from build123d import *

# Parameters (mm, degrees)
SKETCH3_W           = 241.3
SKETCH3_H           = 241.3
SKETCH3_R           = 4.25
BOSS_EXTRUDE1_DEPTH = 12.7
SKETCH4_R           = 7.9375
CUT_EXTRUDE1_DEPTH  = 172.096858533
FILLET1_R           = 12.7
SKETCH5_R           = 7.9375
SKETCH5_R_2         = 10.99947
BOSS_EXTRUDE2_DEPTH = 25.4


with BuildPart() as part:
    # Sketch3 → Boss-Extrude1 (new body)
    with BuildSketch(Plane.XY):
        Rectangle(SKETCH3_W, SKETCH3_H)
        with Locations((-60.104076401, 60.208152802)):
            Circle(SKETCH3_R, mode=Mode.SUBTRACT)
        with Locations((60.104076401, 60.208152802)):
            Circle(SKETCH3_R, mode=Mode.SUBTRACT)
        with Locations((60.104076401, -60)):
            Circle(SKETCH3_R, mode=Mode.SUBTRACT)
        with Locations((-60.104076401, -60)):
            Circle(SKETCH3_R, mode=Mode.SUBTRACT)
    extrude(amount=BOSS_EXTRUDE1_DEPTH)

    # Sketch4 → Cut-Extrude1 (cut, through all)
    with BuildSketch(Plane.XY.offset(12.7)):
        with Locations((-101.6, -101.6)):
            Circle(SKETCH4_R)
        with Locations((101.6, -101.6)):
            Circle(SKETCH4_R)
        with Locations((101.6, 101.6)):
            Circle(SKETCH4_R)
        with Locations((-101.6, 101.6)):
            Circle(SKETCH4_R)
    extrude(amount=-CUT_EXTRUDE1_DEPTH, mode=Mode.SUBTRACT)

    # Fillet1
    fillet1_edges = [part.edges().sort_by_distance(p)[0] for p in [
        (-120.65, 120.65, 6.35),
        (120.65, 120.65, 6.35),
        (120.65, -120.65, 6.35),
        (-120.65, -120.65, 6.35),
    ]]
    fillet(fillet1_edges, radius=FILLET1_R)

    # Sketch5 → Boss-Extrude2 (add)
    with BuildSketch(Plane(origin=(0, 0, 0), x_dir=(-1, 0, 0), z_dir=(0, 0, -1))):
        with BuildLine():
            Line((-107.95, -120.65), (107.95, -120.65))
            ThreePointArc((107.95, -120.65), (116.930256121, -116.930256121), (120.65, -107.95))
            Line((120.65, -107.95), (120.65, 107.95))
            ThreePointArc((120.65, 107.95), (116.930256121, 116.930256121), (107.95, 120.65))
            Line((107.95, 120.65), (-107.95, 120.65))
            ThreePointArc((-107.95, 120.65), (-116.930256121, 116.930256121), (-120.65, 107.95))
            Line((-120.65, 107.95), (-120.65, -107.95))
            ThreePointArc((-120.65, -107.95), (-116.930256121, -116.930256121), (-107.95, -120.65))
        make_face()
        with Locations(Location((101.6, 101.6, 0), (0, 0, 180))):
            Circle(SKETCH5_R, mode=Mode.SUBTRACT)
        with Locations(Location((101.6, -101.6, 0), (0, 0, 180))):
            Circle(SKETCH5_R, mode=Mode.SUBTRACT)
        with Locations(Location((-101.6, -101.6, 0), (0, 0, 180))):
            Circle(SKETCH5_R, mode=Mode.SUBTRACT)
        with Locations(Location((-101.6, 101.6, 0), (0, 0, 180))):
            Circle(SKETCH5_R, mode=Mode.SUBTRACT)
        with Locations((-60.104076401, 60.208152802)):
            Circle(SKETCH5_R_2, mode=Mode.SUBTRACT)
        with Locations((60.104076401, 60.208152802)):
            Circle(SKETCH5_R_2, mode=Mode.SUBTRACT)
        with Locations((60.104076401, -60)):
            Circle(SKETCH5_R_2, mode=Mode.SUBTRACT)
        with Locations((-60.104076401, -60)):
            Circle(SKETCH5_R_2, mode=Mode.SUBTRACT)
    extrude(amount=BOSS_EXTRUDE2_DEPTH)


solid = part.part
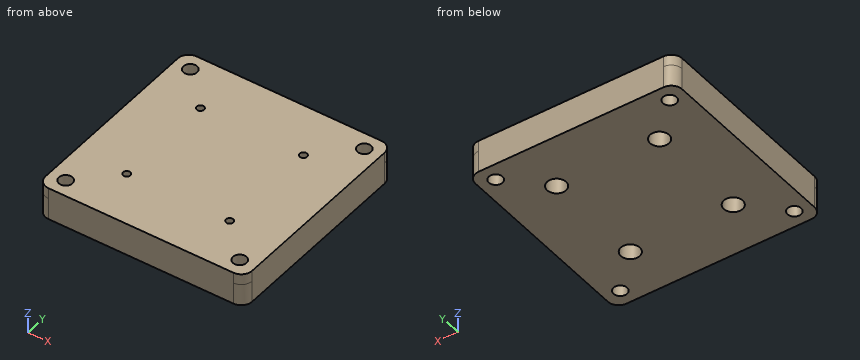
Can you work these out from the model? Positions are in its coordinate system, mm. Give positions to 0.01 mm unless a question says otherwise; leave off trailing zeros. Loops run counter-clockwise (first coordinate to the right, second up) from the corner with the lowest first, then second, coordinate; pieces in that order, holes last. Notation, with made-up numbers: M 80.5,-19 L 138.5,-19 A14 cw 138.5,-3 Z; hole C -18.75,22.25 d2. An arc over 180 degrees is marked long. One line per item, written item: value.
1) Imagine slicing it at A-A on y = -101.6. Write out the boundary of the cut face in (x, z), and give its area (3 significant figures).
Geometry check:
outline: M -120.65,-25.4 L -109.54,-25.4 L -109.54,12.7 L -120.65,12.7 Z; M -93.66,-25.4 L 93.66,-25.4 L 93.66,12.7 L -93.66,12.7 Z; M 109.54,-25.4 L 120.65,-25.4 L 120.65,12.7 L 109.54,12.7 Z
area: 7,980 mm²
2) I'm going to push a flat-ended pin straight in: pin 1 (6.5 mm diameter, centred on x = -60.5, y = 61.5, fed in from -Z). Where does the tip first touch, or does it pass through?
Geometry check:
pin 1: stops at z = 0
3) Please list where these lines run through material, in increasing order: line 1 (Y direction, x = 101.6, z = -15); line 2 (Y direction, x = 101, z = -3); line 3 (X direction, y = -65.5, z = -15).
Geometry check:
line 1: y = -120.65 to -109.54, -93.66 to 93.66, 109.54 to 120.65
line 2: y = -120.65 to -109.51, -93.69 to 93.69, 109.51 to 120.65
line 3: x = -120.65 to -69.63, -50.58 to 50.58, 69.63 to 120.65
4) Imagine slicing it at C-C on z = 8.5. Count the separate pieces of the cut face and the enclosed holes in it, and give its area (3 significant figures).
Geometry check:
separate pieces: 1
enclosed holes: 8
area: 57,100 mm²
